Geometry check sheet. Reference: the model listing, model coordinates, mm. Face numbers are marked on the shaded views. A direction names the side the tool comes from. Coordinates: 2 decimals unless noted, no trailing zeros. Loops run counter-clockwise (first coordinate to the right, second up) from the corner with the lowest first, then second, coordinate; pieces in that order, holes last.
from build123d import *

# Parameters (mm, degrees)
BOSS_EXTRUDE1_DEPTH   = 25.4
SKETCH3_R             = 19.05
SKETCH3_R_2           = 3.175
BOSS_EXTRUDE2_DEPTH   = 6.35
CUT_EXTRUDE1_DEPTH    = 25.4
BOSS_EXTRUDE3_START   = -0.79375
BOSS_EXTRUDE3_DEPTH   = 4.7625
BODY_MOVE_COPY1_ANGLE = 90


with BuildPart() as part:
    # Sketch2 → Boss-Extrude1 (new body)
    with BuildSketch(Plane.XY):
        Polygon((0, 0), (0, 29.462109876), (63.5, 6.35), (139.7, 6.35), (139.7, 0), align=None)
        Polygon((44.933842059, 6.35), (6.35, 6.35), (6.35, 20.393370033), align=None, mode=Mode.SUBTRACT)
    extrude(amount=BOSS_EXTRUDE1_DEPTH)

    # Sketch3 → Boss-Extrude2 (add)
    with BuildSketch(Plane(origin=(0, 6.35, 0), x_dir=(1, 0, 0), z_dir=(0, 1, 0))):
        with Locations((125.500968343, -12.7)):
            Circle(SKETCH3_R)
        with Locations((125.500968343, -12.7)):
            Circle(SKETCH3_R_2, mode=Mode.SUBTRACT)
    extrude(amount=-BOSS_EXTRUDE2_DEPTH)

    # Sketch3<2> → Cut-Extrude1 (cut)
    with BuildSketch(Plane(origin=(0, 6.35, 0), x_dir=(1, 0, 0), z_dir=(0, 1, 0))):
        with BuildLine():
            ThreePointArc((122.325968343, -12.7), (125.500968343, -15.875), (128.675968343, -12.7))
            Line((128.675968343, -12.7), (122.325968343, -12.7))
        make_face()
        with BuildLine():
            Line((122.325968343, -12.7), (128.675968343, -12.7))
            ThreePointArc((128.675968343, -12.7), (125.500968343, -9.525), (122.325968343, -12.7))
        make_face()
    extrude(amount=-CUT_EXTRUDE1_DEPTH, mode=Mode.SUBTRACT)

    # Sketch3<3> → Boss-Extrude3 (add)
    with BuildSketch(Plane(origin=(0, 6.35, 0), x_dir=(1, 0, 0), z_dir=(0, 1, 0)).offset(BOSS_EXTRUDE3_START)):
        with BuildLine():
            ThreePointArc((122.325968343, -12.7), (125.500968343, -15.875), (128.675968343, -12.7))
            Line((128.675968343, -12.7), (122.325968343, -12.7))
        make_face()
        with BuildLine():
            Line((122.325968343, -12.7), (128.675968343, -12.7))
            ThreePointArc((128.675968343, -12.7), (125.500968343, -9.525), (122.325968343, -12.7))
        make_face()
    extrude(amount=-BOSS_EXTRUDE3_DEPTH)


with BuildPart() as part_1:
    # Body-Move/Copy1: moved
    add(part.part.rotate(Axis((0, 0, 0), (1, 0, 0)), BODY_MOVE_COPY1_ANGLE))


solid = part_1.part
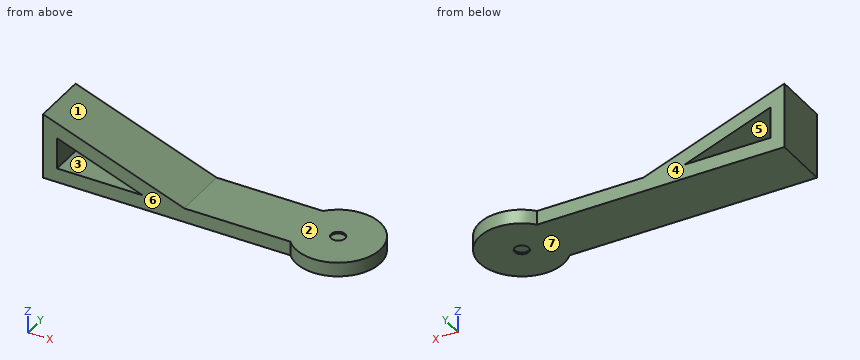
(1) Sectioned sample at B-B on z = 13. Record the cut outline in (x, y).
Findings:
outline: (0, -25.4) - (6.35, -25.4) - (6.35, 0) - (0, 0) - close; (26.66, -25.4) - (45.23, -25.4) - (45.23, 0) - (26.66, 0) - close
(2) Sectioned sample at D-D on y = -2. Record the cut outline in (x, z), and give its area (3 significant figures).
Findings:
outline: (0, 0) - (141.26, 0) - (141.26, 6.35) - (63.5, 6.35) - (0, 29.46) - close; hole (6.35, 6.35) - (44.93, 6.35) - (6.35, 20.39) - close
area: 1,360 mm2
(3) Access from +Z, -Z, +X, -X, +Y, -Y to the whole of each face (thin tool, end or side, straight path). Record for the marked faces 4, 5, 6 and 7.
Findings:
face 4: +Z, -Z, -X, +Y
face 5: +Y, -Y
face 6: +Z, -Z, -X, -Y
face 7: -Z, +X, -X, +Y, -Y
(4) Sectioned sample at C-C on x = 77. Record the cut outline in (y, z).
Findings:
outline: (-25.4, 0) - (0, 0) - (0, 6.35) - (-25.4, 6.35) - close
(5) Scan lines: L1, parallel to Y at x = 126, z = 1.75; L2, parallel to Z at x = 33, y = -14; L3, parallel to Z at x = 25, y = -15. Record each from-to range of solid material in increasing order.
Findings:
L1: y = -31.74 to 6.34
L2: z = 0 to 6.35, 10.69 to 17.45
L3: z = 0 to 6.35, 13.61 to 20.36
(6) Sectioned sample at A-A on y = -12.7. Record the cut outline in (x, z), and give its area (3 significant figures).
Findings:
outline: (0, 0) - (122.33, 0) - (122.33, 0.79) - (128.68, 0.79) - (128.68, 0) - (144.55, 0) - (144.55, 6.35) - (128.68, 6.35) - (128.68, 5.56) - (122.33, 5.56) - (122.33, 6.35) - (63.5, 6.35) - (0, 29.46) - close; hole (6.35, 6.35) - (44.93, 6.35) - (6.35, 20.39) - close
area: 1,370 mm2
(7) Gauge pin test, flat ends, axial feed: pin 1 Ø3 at (y, z) = (-10.5, 3.5) entering from +X; pin 2 Ø8 at (x, z) = (31, 6) entering from -Y; pin 3 Ø10 at (x, y) = (125.5, -12.7) entering from -Z; pin 4 Ø4 at (x, y) = (125.5, -12.7) entering from +Z. Record the tip position at first contact, or that the pin passes through.
Findings:
pin 1: stops at x = 144.54
pin 2: stops at y = -25.4
pin 3: stops at z = 0
pin 4: stops at z = 5.56
(8) Draft check along X on the marked faces 1, 2 and 3. Enter one of: +X half, -X half, draft (parallel to the pull), parting line (faces both ways), or undercut.
Findings:
face 1: +X half
face 2: draft
face 3: undercut
